The model under review builds one solid part; all positions refer to its coordinate system, in mm. Face numbers are marked on the shaded views. A direction names the side the tool comes from. Round coordinates to 2 decimals unless told otherwise and drop trailing zeros. Order: outer loops, then holes, each group sorted by start corner. A loop starts at its lowest first (then second) coordinate and runs counter-clockwise, first axis right, second up.
1) Consider section B-B (x = 22). Give the boundary of the cut face in (y, z), then the cut area to 3 significant figures.
2) Clearance check with flat-ended pins moving along their axes: P1, Ø1.5, axis at x = 31, y = 41, coming from the +Z side; P2, Ø1.5, axis at x = 0, z = 76.5, coming from the +Y side; P3, Ø21, axis at y = -49.5, z = 18.5, coming from the +X side. State where each tip first meets the part, or that it passes through.
3) To check wall thickness, follow L1, parallel to X at y = 41.5, z = 21; L2, parallel to Z at x = -34, y = -11; L3, parallel to Y at x = 27.5, z = 20. State the ranges of each line that lie inside material, in increasing order.
4) Consider section A-A (y = 9). Give the boundary of the cut face in (x, z), then the cut area to 3 significant figures.
5) Mouldability with a two-part tool opening along X and no side actions: class the marked faces 1, 2 and 3 as pulls with the +X half, pulls with the -X half, needs draft (parallel to the pull), parting line crosses it, or undercut.
6) Consider section C-C (z = 10). Give the boundary of the cut face in (x, y), then the cut area to 3 significant figures.
7) Consider section D-D (y = -68.5). Give the boundary of the cut face in (x, z).
8) Machinability: for the marked faces 4, 5 and 6, which of the approach directions +Z, -Z, +X, -X, +Y, -Y give a long, thin tool a straight path to every point of the face, cutting with its end or side? Answer none if there is none.
from build123d import *

# Parameters (mm, degrees)
F0_W      = 78.519128263
F0_H      = 116.7847812176
F1_DEPTH  = 25.4
F2_W      = 20.9176447242
F2_H      = 88.5459557176
F3_DEPTH  = 25.401
F4_R      = 10.4588223621
F5_DEPTH  = 25.4
F6_W      = 78.519128263
F6_H      = 98.6174941063
F7_DEPTH  = 25.4
F8_R      = 25.4
F9_W      = 25.4
F9_H      = 42.0989841223
F10_DEPTH = 25.4
F11_DEPTH = 25.4


with BuildPart() as f1:
    # F0 (on Top) → F1 (new body)
    with BuildSketch(Plane.XY):
        Rectangle(F0_W, F0_H)
    extrude(amount=F1_DEPTH)

    # F2 (on face) → F3 (cut, through all)
    with BuildSketch(Plane.XY.offset(25.4)):
        with Locations((0, 58.3923906088)):
            Rectangle(F2_W, F2_H)
    extrude(amount=-F3_DEPTH, mode=Mode.SUBTRACT)

    # F4 (on face) → F5 (cut)
    with BuildSketch(Plane.XY.offset(25.4)):
        with Locations((0, 14.11941275)):
            Circle(F4_R)
    extrude(amount=-F5_DEPTH, mode=Mode.SUBTRACT)

    # F6 (on face) → F7 (join)
    with BuildSketch(Plane.XZ.offset(58.3923906088)):
        with Locations((0, 49.3087470531)):
            Rectangle(F6_W, F6_H)
    extrude(amount=F7_DEPTH)

    # F8
    f8_edges = [f1.edges().sort_by_distance(p)[0] for p in [
        (-39.259564, -71.092391, 98.617494),
        (39.259564, -71.092391, 98.617494),
    ]]
    fillet(f8_edges, radius=F8_R)

    # F9 (on face) → F10 (cut)
    with BuildSketch(Plane.YZ.offset(39.2595641315)):
        with Locations((-71.0923906088, 21.0494920611)):
            Rectangle(F9_W, F9_H)
    extrude(amount=-F10_DEPTH, mode=Mode.SUBTRACT)

    # F11 (cut): a face of the model
    f11_faces = [f1.faces().sort_by_distance(p)[0] for p in [
        (26.5595641315, -58.3923906088, 12.7),
    ]]
    extrude(f11_faces, amount=-F11_DEPTH, mode=Mode.SUBTRACT)


solid = f1.part
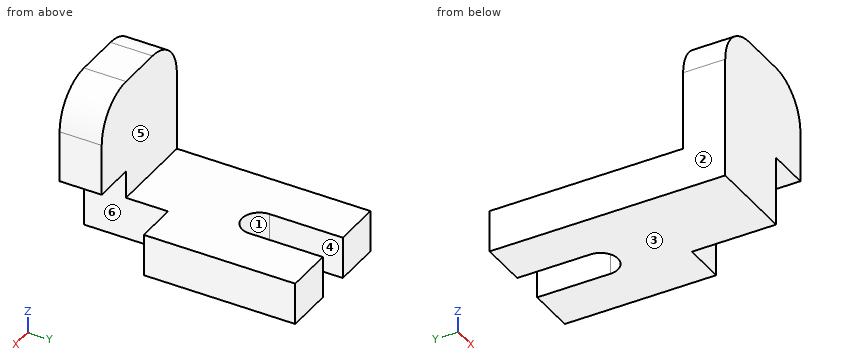
Answer below:
1. outline: (-83.79, 42.1) - (-58.39, 42.1) - (-58.39, 97.28) - (-83.79, 97.28) - close; (-32.99, 0) - (58.39, 0) - (58.39, 25.4) - (-32.99, 25.4) - close
1. area: 3,720 mm2
2. P1: stops at z = 25.4
2. P2: stops at y = -58.39
2. P3: stops at x = 13.86
3. L1: x = -39.26 to -10.46, 10.46 to 39.26
3. L2: z = 0 to 25.4
3. L3: y = -32.99 to 58.39
4. outline: (-39.26, 0) - (-9.12, 0) - (-9.12, 25.4) - (-39.26, 25.4) - close; (9.12, 0) - (39.26, 0) - (39.26, 25.4) - (9.12, 25.4) - close
4. area: 1,530 mm2
5. face 1: undercut
5. face 2: pulls with the -X half
5. face 3: needs draft
6. outline: (-39.26, -83.79) - (13.86, -83.79) - (13.86, -32.99) - (39.26, -32.99) - (39.26, 58.39) - (10.46, 58.39) - (10.46, 14.12) arc R10.46 cw to (-10.46, 14.12) - (-10.46, 58.39) - (-39.26, 58.39) - close
6. area: 8,780 mm2
7. outline: (-39.26, 0) - (13.86, 0) - (13.86, 42.1) - (39.26, 42.1) - (39.26, 73.22) arc R25.4 ccw to (13.86, 98.62) - (-13.86, 98.62) arc R25.4 ccw to (-39.26, 73.22) - close
8. face 4: +Z, -Z, +Y
8. face 5: +Z, +X, -X, +Y
8. face 6: -Z, +X, -Y
